Build history of the part. All positions in model axes, mm. A direction names the side the tool comes from. Round coordinates to 2 decimals unless told otherwise and drop trailing zeros. Loops run counter-clockwise (first coordinate to the right, second up) from the corner with the lowest first, then second, coordinate; pieces in that order, holes last. Notation, with made-up numbers: (70, 47) - (118, 47) arc R6 cw to (118, 58) - close; hole circle Ø8 at (45.25, 86.5). An arc over 180 degrees is marked (long way). Use one line per item in the form item = value. Start each with the question number.
Q1. Pin check, flat tips, straight feed: pin 1 (8 mm diameter, centred on y = -4, z = -3, fed in from +X); pin 2 (10 mm diameter, centred on x = -54, y = -13.5, fed in from +Z); pin 3 (3 mm diameter, centred on x = -4.5, z = -2, fed in from -Y); pin 4 (7 mm diameter, centred on x = -80, z = -5, fed in from +Y). Stop position of each tip, or through.
Q2. 3-axis set-ups, long thin cutter, end or side, ignore diameter. For faces 1 (the face through (-39.8, 0.2, -10)), 2 (the face through (-77, 20, -8)), 3 (the face through (-40, 0, -5)), 4 (the face through (-39.8, 0.2, 0)): which of +Z, -Z, +X, -X, +Y, -Y reach the whole face in a straight line?
Q3. Mould opens along X. For faces 5 (the face through (-77, -20, -8)), 6 (the face through (-53.698, 15.847, -4.93)) say: released by +X, released by -X, zero draft, split by the parting line, or undercut.
Q4. Saw through at B-B (x = 0). Give the cut face in (y, z).
Q5. Saw through at D-D (x = -52.5). Give the cut face in (y, z).
Q6. Drill centre lines: line 1 (Y direction, x = 0, z = -6); line 2 (X direction, y = 2.5, z = -4.75); line 3 (Z direction, x = -80, y = -4). Where is each one in solid material? Low to high.
Q7. Saw through at C-C (y = 22). Give the cut face in (x, z), then the cut area to 3 significant figures.
Q8. Saw through at A-A (y = 0). Give the cut face in (x, z), then the cut area to 3 significant figures.
```python
from build123d import *

# Parameters (mm, degrees)
F2_R     = 35
F2_R_2   = 29.9999993294
F3_DEPTH = 15
F4_R     = 7.5
F4_R_2   = 3.75
F5_DEPTH = 20
F6_DEPTH = 10


with BuildPart() as f3:
    # F2 (on offset) → F3 (new body)
    with BuildSketch(Plane.XY.offset(2.5)):
        Circle(F2_R)
        Circle(F2_R_2, mode=Mode.SUBTRACT)
    extrude(amount=-F3_DEPTH)



with BuildPart() as f5:
    # F4 (on Front) → F5 (new body, symmetric)
    with BuildSketch(Plane.XZ):
        with Locations((-80, -5)):
            Circle(F4_R)
        with Locations((-80, -5)):
            Circle(F4_R_2, mode=Mode.SUBTRACT)
    extrude(amount=F5_DEPTH, both=True)


with BuildPart() as f3_1:
    add(f3.part)

    add(f5.part)  # F6 merges F5
    # F0 (on Top) → F6 (join)
    with BuildSketch(Plane.XY):
        with BuildLine():
            ThreePointArc((-9.6227058053, -33.6512040347), (-35, 0), (-9.6227058053, 33.6512040347))
            Line((-9.6227058053, 33.6512040347), (-74.41, 15.125))
            Line((-74.41, 15.125), (-74.41, -15.125))
            Line((-74.41, -15.125), (-9.6227058053, -33.6512040347))
        make_face()
        with BuildLine():
            ThreePointArc((-39.4029946243, 19.9349947238), (-36.8231138473, 19.164822755), (-36.4382668191, 16.5000821579))
            ThreePointArc((-36.4382668191, 16.5000821579), (-40, 0), (-36.4382668191, -16.5000821579))
            ThreePointArc((-36.4382668191, -16.5000821579), (-36.8231138473, -19.164822755), (-39.4029946243, -19.9349947238))
            Line((-39.4029946243, -19.9349947238), (-67.597336129, -11.8727021118))
            ThreePointArc((-67.597336129, -11.8727021118), (-68.9060386172, -10.9743120453), (-69.41, -9.4690446807))
            Line((-69.41, -9.4690446807), (-69.41, 9.4690446807))
            ThreePointArc((-69.41, 9.4690446807), (-68.9060386172, 10.9743120453), (-67.597336129, 11.8727021118))
            Line((-67.597336129, 11.8727021118), (-39.4029946243, 19.9349947238))
        make_face(mode=Mode.SUBTRACT)
    extrude(amount=-F6_DEPTH)


solid = f3_1.part
```
Report:
q1.pin_1 = 35
q1.pin_2 = 0
q1.pin_3 = -34.87
q1.pin_4 = through
q2.face_1 = -Z
q2.face_2 = +Z, -Z, -X, +Y
q2.face_3 = +Z, -Z
q2.face_4 = +Z
q3.face_5 = zero draft
q3.face_6 = undercut
q4.outline = (-35, -12.5) - (-30, -12.5) - (-30, 2.5) - (-35, 2.5) - close; (30, -12.5) - (35, -12.5) - (35, 2.5) - (30, 2.5) - close
q5.outline = (-21.39, -10) - (-16.19, -10) - (-16.19, 0) - (-21.39, 0) - close; (16.19, -10) - (21.39, -10) - (21.39, 0) - (16.19, 0) - close
q6.line_1 = -35 to -30, 30 to 35
q6.line_2 = -87.5 to -83.74, -76.26 to -69.41, -39.92 to -29.9, 29.9 to 34.91
q6.line_3 = -12.5 to -8.75, -1.25 to 2.5
q7.outline = (-50.37, -10) - (-27.22, -10) - (-27.22, -12.5) - (-20.4, -12.5) - (-20.4, 2.5) - (-27.22, 2.5) - (-27.22, 0) - (-50.37, 0) - close; (20.4, -12.5) - (27.22, -12.5) - (27.22, 2.5) - (20.4, 2.5) - close
q7.area = 436 mm²
q8.outline = (-74.41, -10) - (-69.41, -10) - (-69.41, 0) - (-74.41, 0) arc R7.5 ccw (long way) to start; (-40, -10) - (-35, -10) - (-35, -12.5) - (-30, -12.5) - (-30, 2.5) - (-35, 2.5) - (-35, 0) - (-40, 0) - close; (30, -12.5) - (35, -12.5) - (35, 2.5) - (30, 2.5) - close; hole circle Ø7.5 at (-80, -5)
q8.area = 369 mm²
